Read the model definition and answer for the solid it produces. Units are mm, in the model's axes. Face numbers are marked on the shaded views. A direction names the side the tool comes from. Give positions to 0.01 mm unless a question says otherwise; leave off trailing zeros. Write each loop counter-clockwise with the first axis right and the second up, starting at its lowest first coordinate (ties: lowest second). Pieces come first, ordered by that corner, then holes.
```python
from build123d import *

# Parameters (mm, degrees)
F1_DEPTH = 2
F3_DEPTH = 25
F5_DEPTH = 7
F7_DEPTH = 2
F8_SIZE2 = 0.5773502692
F8_SIZE  = 1
F9_R     = 2


with BuildPart() as f1:
    # F0 (on Top) → F1 (new body)
    with BuildSketch(Plane.XY):
        Polygon((0, 32), (0, 0), (32, 0), align=None)
    extrude(amount=F1_DEPTH)

    # F2 (on face) → F3 (cut)
    with BuildSketch(Plane.XY.offset(2)):
        with BuildLine():
            Line((11.0502525317, 20.9497474683), (7.1611652352, 17.0606601718))
            ThreePointArc((7.1611652352, 17.0606601718), (7.1611652352, 7.1611652352), (17.0606601718, 7.1611652352))
            Line((17.0606601718, 7.1611652352), (20.9497474683, 11.0502525317))
            Line((20.9497474683, 11.0502525317), (11.0502525317, 20.9497474683))
        make_face()
    extrude(amount=-F3_DEPTH, mode=Mode.SUBTRACT)

    # F4 (on face) → F5 (join)
    with BuildSketch(Plane.XY.offset(2)):
        Polygon((0, 32), (0, 0), (32, 0), (30, 2), (2, 2), (2, 30), align=None)
    extrude(amount=F5_DEPTH)

    # F6 (on face) → F7 (join)
    with BuildSketch(Plane.XY.offset(9)):
        Polygon((0, 32), (0, 0), (32, 0), (30, 2), (24, 8), (12, 8), (8, 12), (8, 24), (2, 30), align=None)
    extrude(amount=F7_DEPTH)

    # F8
    f8_edges = [f1.edges().sort_by_distance(p)[0] for p in [
        (10, 10, 9),
    ]]
    chamfer(f8_edges, length=F8_SIZE, length2=F8_SIZE2)

    # F9
    f9_edges = [f1.edges().sort_by_distance(p)[0] for p in [
        (0, 0, 5.5),
    ]]
    fillet(f9_edges, radius=F9_R)


solid = f1.part
```
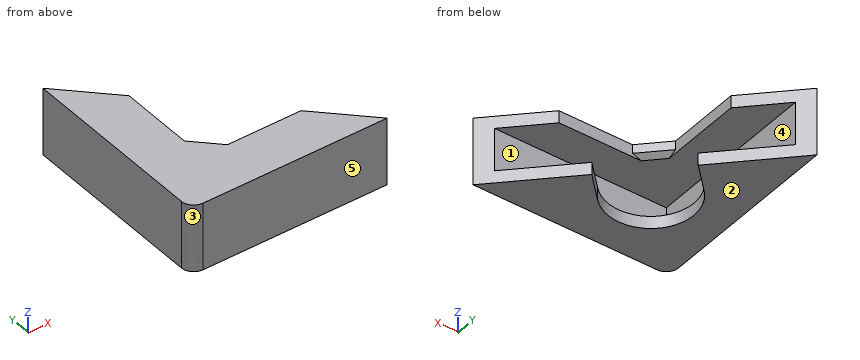
Item 1: Section B-B (z = 1.5) is taken. Write down the section's boundary in (x, y).
Result set:
outline: (0, 2) arc R2 ccw to (2, 0) - (32, 0) - (20.95, 11.05) - (17.06, 7.16) arc R7 cw to (7.16, 17.06) - (11.05, 20.95) - (0, 32) - close
Item 2: Section D-D (y = 6) is taken. Write down the section's boundary in (x, z), and give its area (3 significant figures).
Result set:
outline: (0, 0) - (8.7, 0) - (8.7, 2) - (2, 2) - (2, 9) - (26, 9) - (26, 11) - (0, 11) - close; (15.53, 0) - (26, 0) - (26, 2) - (15.53, 2) - close
area: 104 mm2
Item 3: Find the intervals of material crossed by line 1 along Z through (x, y) = (7.5, 18); line 2 along Y through (x, z) = (29.5, 7.75), in increasing order.
Result set:
line 1: z = 0 to 2, 9 to 11
line 2: y = 0 to 2
Item 4: Section C-C (y = 26.5) is taken. Write down the section's boundary in (x, z).
Result set:
outline: (0, 0) - (5.5, 0) - (5.5, 2) - (2, 2) - (2, 9) - (5.5, 9) - (5.5, 11) - (0, 11) - close
Item 5: Determine the mould class of the marked faces 1, 2 and 3 for opening direction Y: pulls with the +Y half, pulls with the -Y half, needs draft (parallel to the pull), parting line crosses it, or undercut.
Result set:
face 1: pulls with the +Y half
face 2: needs draft
face 3: pulls with the -Y half
Item 6: Each of these flat-tipped pins is pushed along its axis until it touches: pin 1 Ø14 at (x, y) = (12, 10.5) entering from +Z; pin 2 Ø4 at (y, z) = (26, 6) entering from +X; pin 3 Ø1.5 at (y, z) = (23.5, 2.5) entering from +X; pin 4 Ø0.6 at (x, z) = (20, 10) entering from +Y. Where does it stop, or does it pass through?
Result set:
pin 1: stops at z = 11
pin 2: stops at x = 2
pin 3: stops at x = 9.06
pin 4: stops at y = 8
Item 7: Section A-A (x = 5.5) is taken. Write down the section's boundary in (y, z), and give its area (3 significant figures).
Result set:
outline: (0, 0) - (9.81, 0) - (9.81, 2) - (2, 2) - (2, 9) - (26.5, 9) - (26.5, 11) - (0, 11) - close; (14.41, 0) - (26.5, 0) - (26.5, 2) - (14.41, 2) - close
area: 111 mm2
Item 8: Which of the six approach directions +Z, -Z, +X, -X, +Y, -Y give full straight-line access (tool end or side, diameter ignored) to the marked faces 4 and 5?
Result set:
face 4: +X, +Y
face 5: +Z, -Z, +X, -X, -Y
